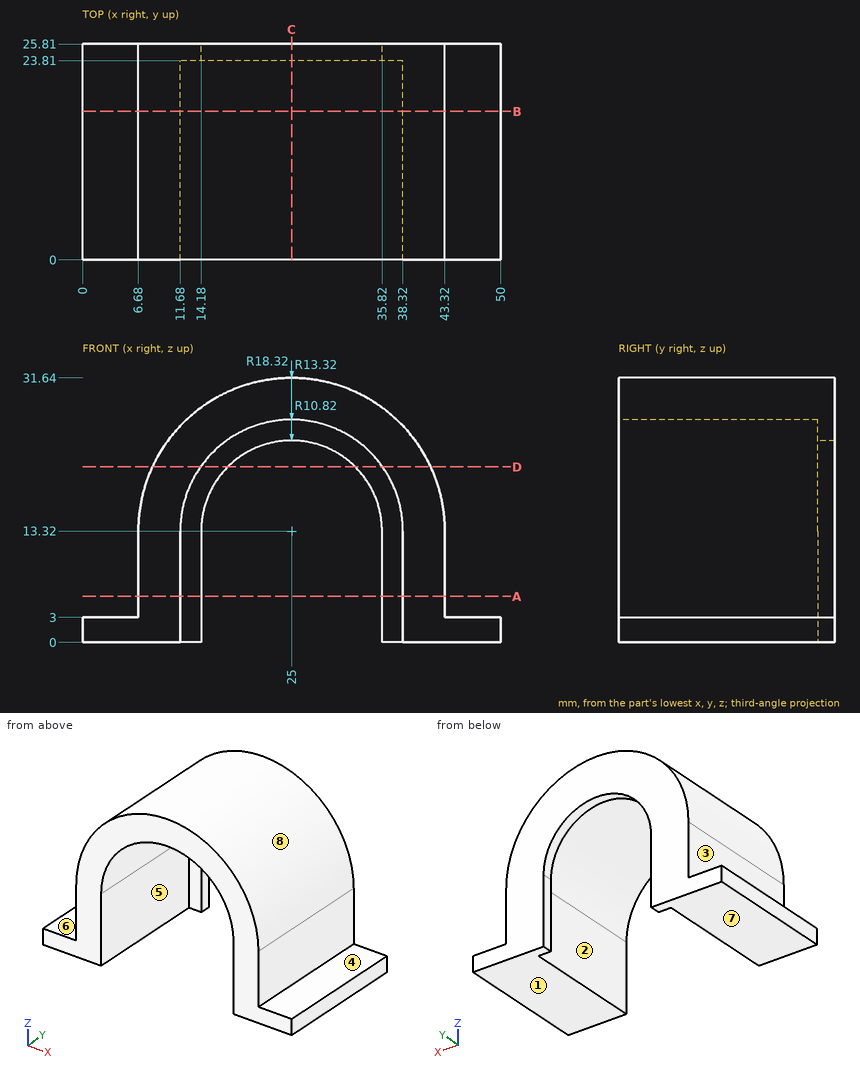
Here's the drawing with two shaded views (mm, measured from the low corner). I have some questions. A direction names the side the tool comes from. Coordinates: 2 decimals unless noted, no trailing zeros. Loops run counter-clockwise (first coordinate to the right, second up) from the corner with the lowest first, then second, coordinate; pieces in that order, holes last. Notation, with made-up numbers: M 84,88.25 L 90,88.25 A13 ccw 90,108.25 Z; hole C 67,87.25 d7. An arc over 180 degrees is marked long. Put each result on its own line as item: value. Start each with the question number.
(1) We'd pull the mould along X, two halves only. Please class the marked faces 1, 2 and 3: +X half, -X half, draft (parallel to the pull), parting line (faces both ways), or undercut.
(2) Which directions (+Z, -Z, +X, -X, +Y, -Y) give clear straight access to the entire face, cutting with the end or side of a thin tool? Please do the marked faces 4, 5, 6, 7 and 8.
(3) Imagine slicing it at B-B on y = 17.75. List the corners of the cut face in (x, z) for me.
(4) Will these pins go through, and if not, where does the flat tip stop? pin 1 Ø4 at (x, y) = (40.5, 10) entering from +Z; pin 2 Ø1 at (y, z) = (8.5, 6) entering from -X; pin 3 Ø10 at (x, z) = (21, 20.5) entering from -Y.
(5) Imagine slicing it at D-D on z = 21. List the corners of the cut face in (x, y) for me, and give its area (3 significant figures).
(6) Imagine slicing it at C-C on x = 25. List the corners of the cut face in (y, z) for me.
(7) Imagine slicing it at A-A on z = 5.5. List the corners of the cut face in (x, y) for me.
(8) I need wall thicknesses on probe 1 along X at (y, z) = (14.5, 5.5); probe 2 along X at (y, z) = (2, 24.5); probe 3 along Z at (x, y) = (24.5, 19.75). Which ranges of each line are inside material? Lowest first, please.
Worked answers:
1. face 1: draft
1. face 2: undercut
1. face 3: -X half
2. face 4: +Z, +X, +Y, -Y
2. face 5: -Z, -Y
2. face 6: +Z, -X, +Y, -Y
2. face 7: -Z, +X, -X, +Y, -Y
2. face 8: +Z, +Y, -Y
3. outline: M 0,0 L 11.68,0 L 11.68,13.32 A13.32 cw 38.32,13.32 L 38.32,0 L 50,0 L 50,3 L 43.32,3 L 43.32,13.32 A18.32 ccw 6.68,13.32 L 6.68,3 L 0,3 Z
4. pin 1: stops at z = 25.7
4. pin 2: stops at x = 6.68
4. pin 3: stops at y = 23.81
5. outline: M 8.37,0 L 14.12,0 L 14.12,23.81 L 17.38,23.81 L 17.38,25.81 L 8.37,25.81 Z; M 32.62,23.81 L 35.88,23.81 L 35.88,0 L 41.63,0 L 41.63,25.81 L 32.62,25.81 Z
5. area: 310 mm2
6. outline: M 0,26.64 L 23.81,26.64 L 23.81,24.14 L 25.81,24.14 L 25.81,31.64 L 0,31.64 Z
7. outline: M 6.68,0 L 11.68,0 L 11.68,23.81 L 14.18,23.81 L 14.18,25.81 L 6.68,25.81 Z; M 35.82,23.81 L 38.32,23.81 L 38.32,0 L 43.32,0 L 43.32,25.81 L 35.82,25.81 Z
8. probe 1: x = 6.68 to 11.68, 38.32 to 43.32
8. probe 2: x = 10.49 to 17.76, 32.24 to 39.51
8. probe 3: z = 26.63 to 31.63
